Autodesk Inventor part; units mm, degrees
ref_plane "YZ Plane" through (0, 0, 0) normal (1, 0, 0) x (0, 1, 0)
ref_plane "XZ Plane" through (0, 0, 0) normal (0, 1, 0) x (-1, 0, 0)
ref_plane "XY Plane" through (0, 0, 0) normal (0, 0, 1) x (1, 0, 0)
sketch "Sketch1" plane through (0, 0, 0) normal (1, 0, 0) x (0, 1, 0)
  line L0 (0, 0) -> (31.75, 0)
  line L1 (31.75, 0) -> (31.75, -31.75)
  line L2 (31.75, -31.75) -> (0, -31.75)
  line L3 (0, -31.75) -> (0, 0)
  line L4 (29.75, -29.75) -> (29.75, -2)
  line L5 (29.75, -2) -> (2, -2)
  line L6 (2, -2) -> (2, -29.75)
  line L7 (2, -29.75) -> (29.75, -29.75)
  dimension "d0" = 31.75
  dimension "d1" = 31.75
  dimension "d2" = 2
extrude "Extrusion1" add sketch "Sketch1" along normal blind 600
sketch "Sketch2" plane through (0, 31.75, 0) normal (0, 1, 0) x (1, 0, 0)
  line L0 (0, 0) -> (600, 0)
  line L1 (600, 0) -> (400, 0)
  line L2 (0, 0) -> (400, 0)
  line L3 (0, 0) -> (400, 0)
  line L4 (0, 0) -> (200, 0)
  line L5 (0, 31.75) -> (0, 0)
  line L6 (0, 0) -> (600, 0)
  line L7 (600, 31.75) -> (600, 0)
  line L8 (0, 31.75) -> (600, 31.75)
  circle A0 centre (286.75, 15.875) radius 6
  circle A1 centre (113.25, 15.875) radius 6
  circle A2 centre (175, 15.875) radius 6
  circle A3 centre (225, 15.875) radius 6
  dimension "d5" = 200
  dimension "d6" = 200
  dimension "d7" = 12
  dimension "d8" = 86.75
  dimension "d9" = 12
  dimension "d10" = 86.75
  dimension "d11" = 12
  dimension "d12" = 61.75
  dimension "d13" = 12
  dimension "d14" = 61.75
extrude "Extrusion2" cut sketch "Sketch2" against normal through all contours A0 | A1 | A2 | A3
sketch "Sketch3" plane through (0, 0, -31.75) normal (0, 0, -1) x (-1, 0, 0)
  line L0 (-600, 0) -> (-550, 0)
  line L1 (0, 0) -> (-600, 0)
  line L2 (0, 0) -> (0, 31.75)
  line L3 (0, 31.75) -> (-600, 31.75)
  line L4 (-600, 0) -> (-600, 31.75)
  line L5 (0, 0) -> (-600, 0)
  circle A0 centre (-550, 15.875) radius 6
  circle A1 centre (-488.25, 15.875) radius 6
  dimension "d17" = 50
  dimension "d19" = 12
  dimension "d20" = 12
  dimension "d21" = 61.75
extrude "Extrusion3" cut sketch "Sketch3" against normal through all contours A0 | A1
sketch "Sketch4" plane through (0, 0, -31.75) normal (0, 0, -1) x (-1, 0, 0)
  circle A0 centre (-296, 15.875) radius 6
  circle A1 centre (-488.25, 15.875) radius 6
  circle A2 centre (-234.25, 15.875) radius 6
  point P0 (0, 0)
  dimension "d24" = 12
  dimension "d25" = 180.25
  dimension "d28" = 12
  dimension "d29" = 61.75
extrude "Extrusion4" cut sketch "Sketch4" against normal through all contours A0 | A2
properties part number "Base_Fija_Acero"
Here's how the part is built. I have some questions about the finished solid (model axes, mm). A direction names the side the tool comes from. Give positions to 0.01 mm unless a question says otherwise; leave off trailing zeros. Order: outer loops, then holes, each group sorted by start corner. A loop starts at its lowest first (then second) coordinate and runs counter-clockwise, first axis right, second up. Notation, with made-up numbers: (70.5, 72.5) -> (83.5, 72.5) arc R20 ccw to (83.5, 104.5) -> close; hole circle Ø2 at (17.25, 65). An arc over 180 degrees is marked (long way). Use CSV: the item, a comma, the result in double quotes. Start each with the question number.
Item 1: Suppose I cut it at B-B (x = 154.5). List the corners of the cut face in (y, z) for me, and give its area (3 significant figures).
Item 2: If I drill on probe 1 along Z at (x, y) = (330.5, 4.5); probe 2 along Y at (x, z) = (55.5, -8.5); probe 3 along Z at (x, y) = (286.75, 30.6) (3 decimals), over which ranges is the centre line in solid material (lowest first)? Write a range as [from, to].
Item 3: I'm going to push a flat-ended pin straight in: P1, Ø10, axis at y = 24.5, z = -19.5, coming from the +X side. Where does the tip first touch, or does it pass through?
Item 4: Suppose I cut it at A-A (x = 550). List the corners of the cut face in (y, z) for me (3 decimals).
Item 5: Thinking about a two-plate mould opening in X: for faces 1 (the flat face through (600, 30, -16)), 2 (the cylindrical face through (292.47, 30.76, -17.68)), 3 (the flat face through (296, 29.75, -16)), which applies, pulls with the +X half, pulls with the -X half, needs draft (parallel to the pull), parting line crosses it, or undercut?
Item 6: On a 3-axis mill with a long thin cutter (end or side, diameter ignored), from which of +Z, -Z, +X, -X, +Y, -Y can I reach the whole of each face in a straight line? I mean faces 4 (the cylindrical face through (230.72, 30.76, -17.68)), 5 (the flat face through (296, 2, -16)). Say none if no direction works.
Answer block:
1,outline,"(0, -31.75) -> (31.75, -31.75) -> (31.75, 0) -> (0, 0) -> close; hole (2, -29.75) -> (29.75, -29.75) -> (29.75, -2) -> (2, -2) -> close"
1,area,"238 mm^2"
2,probe 1,"z = [-31.75, -29.75], [-2, 0]"
2,probe 2,"y = [0, 2], [29.75, 31.75]"
2,probe 3,"z = [-31.75, -21.875], [-9.875, 0]"
3,P1,"passes through"
4,outline,"(0, -31.75) -> (9.875, -31.75) -> (9.875, -29.75) -> (2, -29.75) -> (2, -2) -> (9.875, -2) -> (9.875, 0) -> (0, 0) -> close; (21.875, -31.75) -> (31.75, -31.75) -> (31.75, 0) -> (21.875, 0) -> (21.875, -2) -> (29.75, -2) -> (29.75, -29.75) -> (21.875, -29.75) -> close"
5,face 1,"pulls with the +X half"
5,face 2,"undercut"
5,face 3,"needs draft"
6,face 4,"+Y, -Y"
6,face 5,"+X, -X"
